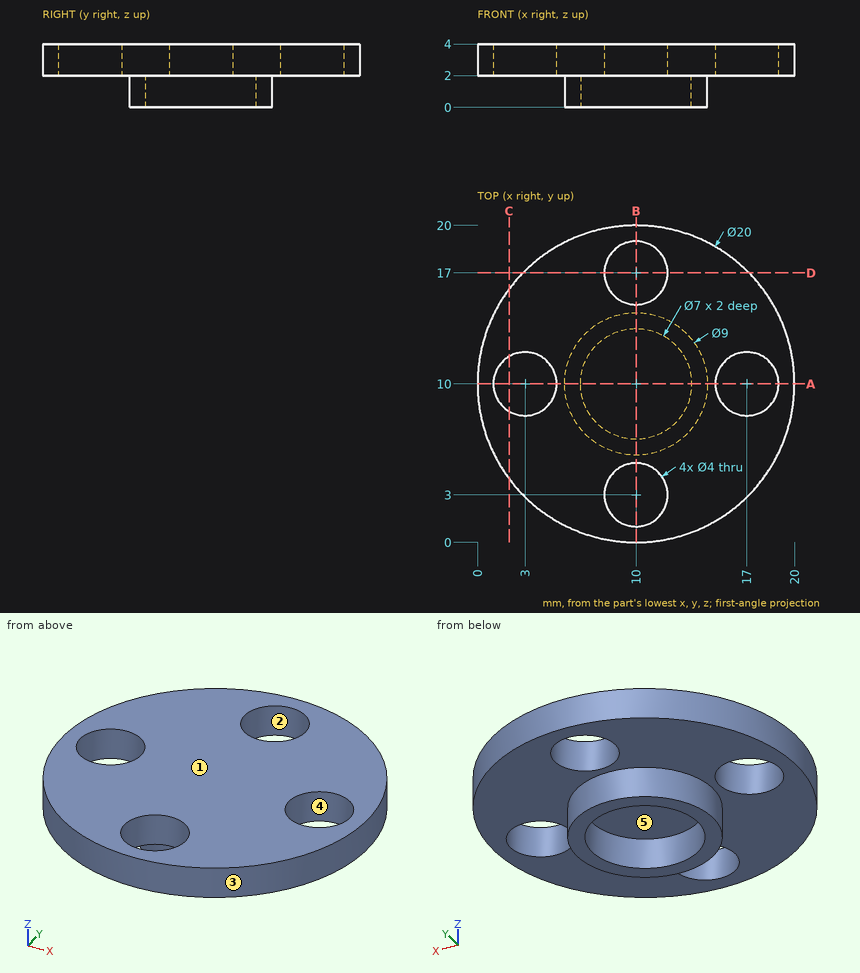
Check sheet for the drawn part. Datum: minimum x, y, z corner. Units: mm. A direction names the side the tool comes from. Coordinates: 2 decimals unless noted, no trailing zeros. Write each loop counter-clockwise with the first axis right and the second up, starting at its lowest first coordinate (ties: lowest second). Pieces come first, ordered by that corner, then holes. Notation, with made-up numbers: M 79.25,0.25 L 90.25,0.25 A29 ccw 90.25,27.25 Z; hole C 26.5,-16 d8. An arc over 180 degrees is marked long. Use a Markdown table: item, result.
Q1. Go/stop test with flat-tipped pins: P1, Ø1.5, axis at y = 8.5, z = 2.5, coming from the -X side; P2, Ø10, axis at x = 2, y = 3.5, coming from the -Z side; P3, Ø1, axis at x = 12.5, z = 3, coming from the -Y side; P4, Ø3, axis at x = 10, y = 3, coming from the -Z side. Record where each tip stops, or that it passes through.
Reply:
| item | result |
|---|---|
| P1 | stops at x = 0.03 |
| P2 | stops at z = 2 |
| P3 | stops at y = 0.2 |
| P4 | passes through |
Q2. Thickness scan on line 1 (Y direction, x = 10, z = 3.45); line 2 (Y direction, x = 10, z = 0.8); line 3 (Z direction, x = 14.25, y = 1.25). Record the ranges inside material, lowest first.
Reply:
| item | result |
|---|---|
| line 1 | y = 0 to 1, 5 to 15, 19 to 20 |
| line 2 | y = 5.5 to 6.5, 13.5 to 14.5 |
| line 3 | z = 2 to 4 |
Q3. Draft check along X on the marked faces 1, 2 and 3. Enter one of: +X half, -X half, draft (parallel to the pull), parting line (faces both ways), or undercut.
Reply:
| item | result |
|---|---|
| face 1 | draft |
| face 2 | undercut |
| face 3 | parting line |
Q4. Sectioned sample at A-A, the plane y = 10. Record the boundary of the cut face in (x, z), plus the area to 3 significant figures.
Reply:
| item | result |
|---|---|
| outline | M 0,2 L 1,2 L 1,4 L 0,4 Z; M 5,2 L 5.5,2 L 5.5,0 L 6.5,0 L 6.5,2 L 13.5,2 L 13.5,0 L 14.5,0 L 14.5,2 L 15,2 L 15,4 L 5,4 Z; M 19,2 L 20,2 L 20,4 L 19,4 Z |
| area | 28.0 mm² |
Q5. Set-up check for the marked faces 4 and 5: record each of +Z, -Z, +X, -X, +Y, -Y from which the full face is reachable in a straight line by a thin tool's end or side.
Reply:
| item | result |
|---|---|
| face 4 | +Z, -Z |
| face 5 | -Z |
Q6. Sectioned sample at D-D, the plane y = 17. Record the boundary of the cut face in (x, z), plus the area to 3 significant figures.
Reply:
| item | result |
|---|---|
| outline | M 2.86,2 L 8,2 L 8,4 L 2.86,4 Z; M 12,2 L 17.14,2 L 17.14,4 L 12,4 Z |
| area | 20.6 mm² |
Q7. Sectioned sample at C-C, the plane x = 2. Record the boundary of the cut face in (y, z), plus the area to 3 significant figures.
Reply:
| item | result |
|---|---|
| outline | M 4,2 L 8.27,2 L 8.27,4 L 4,4 Z; M 11.73,2 L 16,2 L 16,4 L 11.73,4 Z |
| area | 17.1 mm² |
